Here's the drawing with two shaded views (mm, measured from the low corner). I have some questions. A direction names the side the tool comes from. Round coordinates to 2 decimals unless told otherwise and drop trailing zeros. Loops run counter-clockwise (first coordinate to the right, second up) from the corner with the lowest first, then second, coordinate; pieces in that order, holes last.
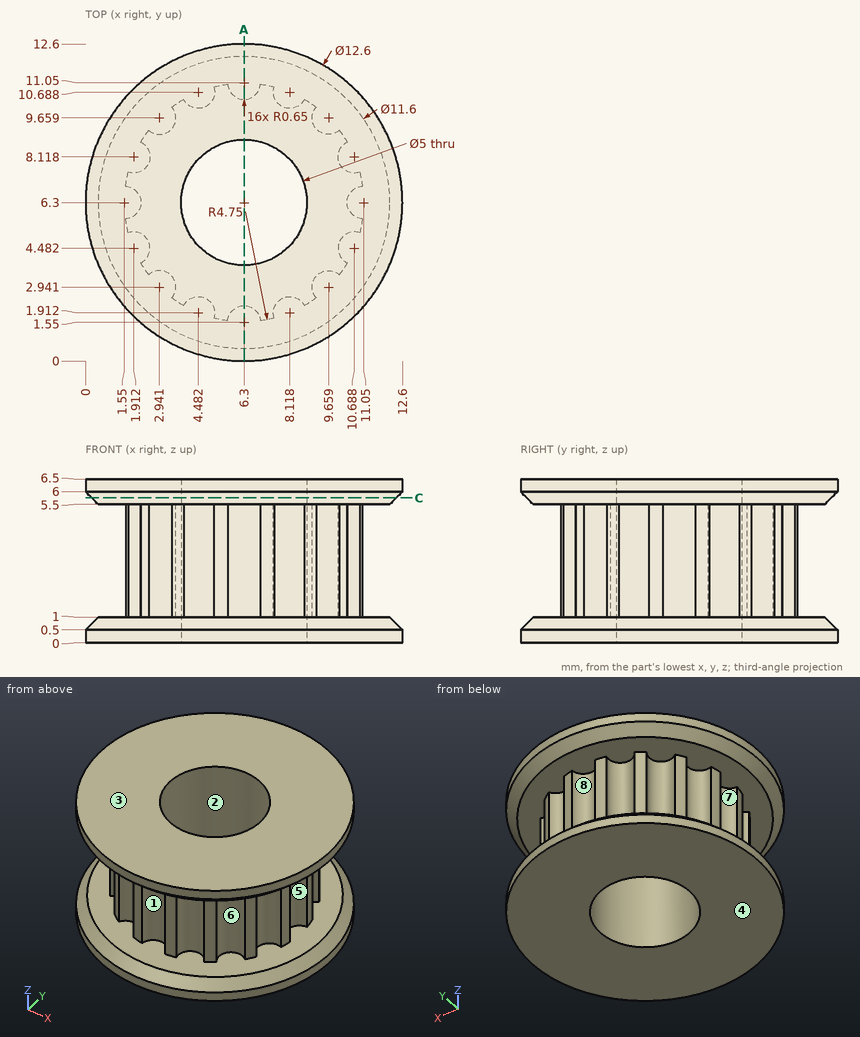
(1) If we section it at C-C, the plane z = 5.75: List the corners of the cut face in (x, y) for me.
Worked answers:
outline: circle Ø12.1 at (6.3, 6.3); hole circle Ø5 at (6.3, 6.3)
(2) For the marked faces 4, 5, 6, 7 and 8, which set-ups out of +Z, -Z, +X, -X, +Y, -Y let a thin tool reach every point of the face, with its end or its side?
Worked answers:
face 4: -Z, +X, -X, +Y, -Y
face 5: +X
face 6: none
face 7: -X
face 8: +Y
(3) Will these pins go through, and if not, where does the flat tip stop? P1, Ø3, axis at y = 3, z = 5, coming from the +X side; P2, Ø6.5, axis at x = 6.3, y = 6.3, coming from the -Z side; P3, Ø1.5, axis at y = 10.5, z = 0.5, coming from the +X side; P4, Ø3, axis at x = 3, z = 3.5, coming from the +Y side.
Worked answers:
P1: stops at x = 12.21
P2: stops at z = 0
P3: stops at x = 11.57
P4: stops at y = 10.4
(4) If I drill on line 1 (Y direction, x = 6.3, z = 5); line 2 (Z direction, x = 4.75, y = 10.25), over which ranges is the centre line in solid material (lowest first)?
Worked answers:
line 1: y = 2.2 to 3.8, 8.8 to 10.4
line 2: z = 0 to 1, 5.5 to 6.5
(5) If we section it at A-A, the plane x = 6.3: List the corners of the cut face in (y, z) for me, then the cut area to 3 significant figures.
Worked answers:
outline: (0, 0) - (3.8, 0) - (3.8, 6.5) - (0, 6.5) - (0, 6) - (0.5, 5.5) - (2.2, 5.5) - (2.2, 1) - (0.5, 1) - (0, 0.5) - close; (8.8, 0) - (12.6, 0) - (12.6, 0.5) - (12.1, 1) - (10.4, 1) - (10.4, 5.5) - (12.1, 5.5) - (12.6, 6) - (12.6, 6.5) - (8.8, 6.5) - close
area: 29.1 mm2
(6) If we mould it in two halves opening along Z, with no side actions, what happens to the marked faces 1, 2 and 3? For each: released by +Z, released by -Z, zero draft, split by the parting line, or undercut.
Worked answers:
face 1: undercut
face 2: zero draft
face 3: released by +Z
